Source: CAD feature listing. Evaluate the final solid. Frame: model axes, mm. A direction names the side the tool comes from. Give positions to 0.01 mm unless a question says otherwise; leave off trailing zeros. Write each loop counter-clockwise with the first axis right and the second up, starting at its lowest first coordinate (ties: lowest second). Pieces come first, ordered by that corner, then holes. Notation, with made-up numbers: (56, 36) -> (104, 36) arc R29 cw to (104, 68) -> close; hole circle Ø10 at (-32.5, 33.25). An arc over 180 degrees is marked (long way). Use a Markdown table: item, result. Add a question column.
```python
from build123d import *

# Parameters (mm, degrees)
F1_DEPTH      = 10
F1_DEPTH_BACK = 10
F2_DEPTH      = 3
F3_DEPTH      = 10
F3_DEPTH_BACK = 10


with BuildPart() as f1:
    # F0 (on Front) → F1 (new body, two sides)
    with BuildSketch(Plane.XZ) as f1_sk:
        Polygon((-9.122807, 39.162219), (-29.122807, 39.162219), (-29.122807, 0), (-9.122807, 0), (116.327327, 105.265161), (148.048821, 131.882655), (128.765193, 154.863988), align=None)
    extrude(amount=F1_DEPTH)
    extrude(f1_sk.sketch, amount=-F1_DEPTH_BACK)

    # F0 (on Front) → F2 (join)
    with BuildSketch(Plane.XZ):
        Polygon((116.327327, 105.265161), (-9.122807, 0), (-9.122807, -104.527941), (28.618485, -82.653101), align=None)
    extrude(amount=F2_DEPTH)

    # F0 (on Front) → F3 (join, two sides)
    with BuildSketch(Plane.XZ) as f3_sk:
        Polygon((28.618485, -82.653101), (-9.122807, -104.527941), (-29.122807, -104.527941), (-29.122807, -124.527941), (9.073851, -124.527941), align=None)
    extrude(amount=F3_DEPTH)
    extrude(f3_sk.sketch, amount=-F3_DEPTH_BACK)


solid = f1.part
```
(1) Mould query, pull axis Z, two halves, no side actions, for faces 1 (the flat face through (-19, 0, 0)), 2 (the flat face through (52, 10, 72)), 3 (the flat face through (-19, 0, 39.162)). Classes: +Z half, -Z half, draft (parallel to the pull), parting line (faces both ways), or undercut.
(2) Material intervals for L1, parallel to Z at x = -12.5, y = -8.5; L2, parallel to Y at x = 40, z = 1; L3, parallel to Z at x = -6.5, y = 4, sorted ascending.
(3) Access query for faces 4 (the flat face through (10.01, -6.45, -93.44)), 5 (the flat face through (10.01, 4.93, -93.44)), 6 (the flat face through (-19, 0, -104.528)), 7 (the flat face through (61, 0, 98)). Directions: +Z, -Z, +X, -X, +Y, -Y. A direction counts if a zero-diameter tool reaches every point of the face in a straight line with its end or side. Return the directions, or none.
(4) Cut plane B-B on y = -7.25. Return the cut outline in (x, z).
(5) Cut plane A-A on x = -17. Return the cut outline in (y, z).
(6) Cut plane D-D on z = 101.5. Return the cut outline in (x, y).
(7) Cut plane C-C on x = 4.5. Return the cut outline in (y, z), then the cut area to 3 significant figures.
(8) First-contact query: pin 1 Ø5 at (x, y) = (84, 5.5) entering from -Z; pin 2 Ø2 at (x, y) = (125, 1.5) entering from +Z; pin 3 Ø2 at (x, z) = (39.5, -25) entering from +Y. Flat tips, straight axial feed; report the tip coordinate or a pass-through.
Output:
| question | item | result |
|---|---|---|
| 1 | face 1 | undercut |
| 1 | face 2 | draft |
| 1 | face 3 | +Z half |
| 2 | L1 | -124.53 to -104.53, 0 to 39.16 |
| 2 | L2 | -3 to 0 |
| 2 | L3 | -124.53 to -103.01, 2.2 to 41.36 |
| 3 | face 4 | -X, -Y |
| 3 | face 5 | -X, +Y |
| 3 | face 6 | -X, +Y, -Y |
| 3 | face 7 | +Z, -X, +Y, -Y |
| 4 | outline | (-29.12, -124.53) -> (9.07, -124.53) -> (28.62, -82.65) -> (-9.12, -104.53) -> (-29.12, -104.53) -> close; (-29.12, 0) -> (-9.12, 0) -> (148.05, 131.88) -> (128.77, 154.86) -> (-9.12, 39.16) -> (-29.12, 39.16) -> close |
| 5 | outline | (-10, -124.53) -> (10, -124.53) -> (10, -104.53) -> (-10, -104.53) -> close; (-10, 0) -> (10, 0) -> (10, 39.16) -> (-10, 39.16) -> close |
| 6 | outline | (65.17, -10) -> (111.84, -10) -> (111.84, -3) -> (114.57, -3) -> (114.57, 0) -> (111.84, 0) -> (111.84, 10) -> (65.17, 10) -> close |
| 7 | outline | (-10, -124.53) -> (10, -124.53) -> (10, -96.63) -> (0, -96.63) -> (0, 11.43) -> (10, 11.43) -> (10, 50.59) -> (-10, 50.59) -> (-10, 11.43) -> (-3, 11.43) -> (-3, -96.63) -> (-10, -96.63) -> close |
| 7 | area | 1,670 mm^2 |
| 8 | pin 1 | z = 76.04 |
| 8 | pin 2 | z = 152.54 |
| 8 | pin 3 | y = 0 |
